Part print with two shaded views. Sizes in mm from the minimum x, y, z corner. Round coordinates to 2 decimals unless told otherwise and drop trailing zeros. Loops run counter-clockwise (first coordinate to the right, second up) from the corner with the lowest first, then second, coordinate; pieces in that order, holes last. Notation, with made-up numbers: (66, -0.5) -> (82, -0.5) arc R32 ccw to (82, 35.5) -> close; hole circle Ø1 at (88, 25). An arc over 180 degrees is marked (long way). Answer as a JSON object with one key per item and string values. Group by question number.
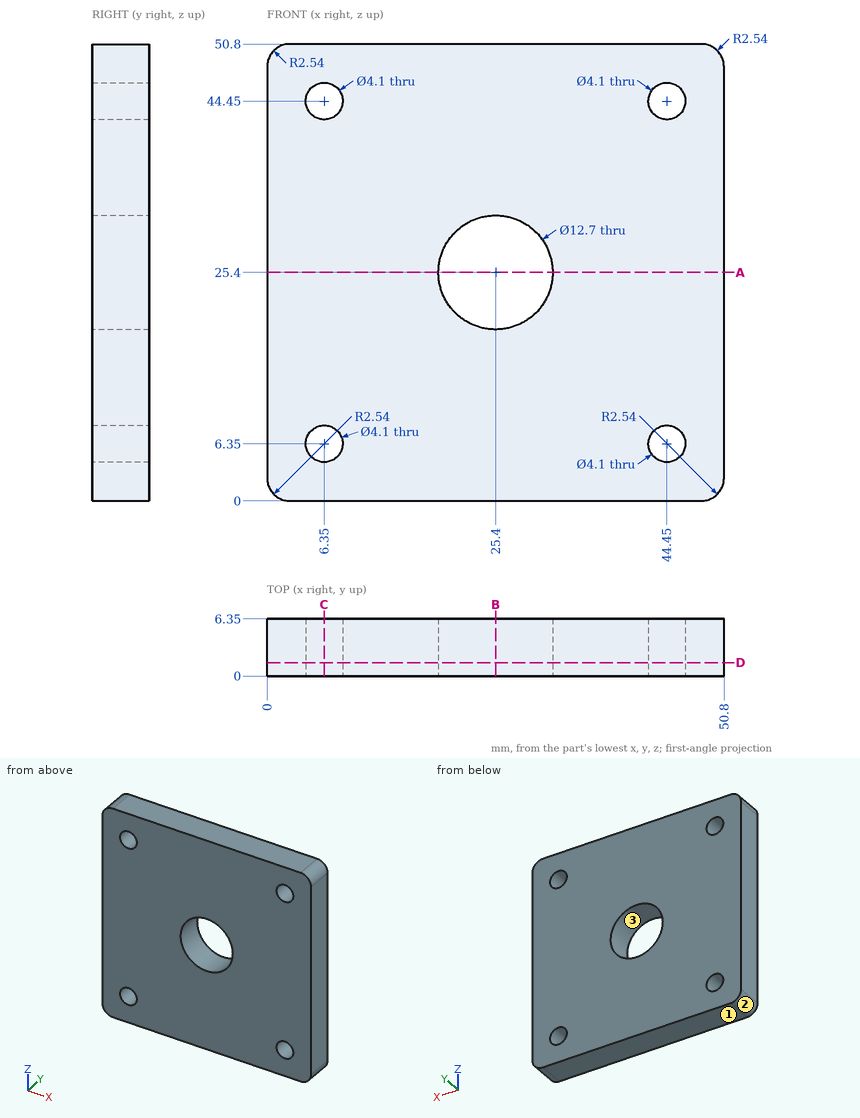
Item 1: Band-saw the part on A-A, the plane z = 25.4. List the corners of the cut face in (x, y).
Item 2: Drill centre lines: line 1 (X direction, y = 1.5, z = 6.35); line 2 (X direction, y = 3.75, z = 25.4); line 3 (Z direction, x = 43.5, y = 3). Where is each one in solid material? Low to high.
Item 3: Band-saw the part on D-D, the plane y = 1.5. List the corners of the cut face in (x, z), plus the area to 3 significant figures.
Item 4: Band-saw the part on B-B, the plane x = 25.4. List the corners of the cut face in (y, z), plus the area to 3 significant figures.
Item 5: Band-saw the part on C-C, the plane x = 6.35. List the corners of the cut face in (y, z), plus the area to 3 significant figures.
Item 6: Two-plate mould, pull along X, no slides. Class the marked faces 1, 2 and 3: pulls with the +X half, pulls with the -X half, needs draft (parallel to the pull), parting line crosses it, or undercut.
Entries:
{
 "1": {"outline": "(0, 0) -> (19.05, 0) -> (19.05, 6.35) -> (0, 6.35) -> close; (31.75, 0) -> (50.8, 0) -> (50.8, 6.35) -> (31.75, 6.35) -> close"},
 "2": {"line 1": "0 to 4.3, 8.4 to 42.4, 46.5 to 50.8", "line 2": "0 to 19.05, 31.75 to 50.8", "line 3": "0 to 4.53, 8.17 to 42.63, 46.27 to 50.8"},
 "3": {"outline": "(0, 2.54) arc R2.54 ccw to (2.54, 0) -> (48.26, 0) arc R2.54 ccw to (50.8, 2.54) -> (50.8, 48.26) arc R2.54 ccw to (48.26, 50.8) -> (2.54, 50.8) arc R2.54 ccw to (0, 48.26) -> close; hole circle Ø4.1 at (6.35, 6.35); hole circle Ø4.1 at (6.35, 44.45); hole circle Ø12.7 at (25.4, 25.4); hole circle Ø4.1 at (44.45, 6.35); hole circle Ø4.1 at (44.45, 44.45)", "area": "2,400 mm²"},
 "4": {"outline": "(0, 0) -> (6.35, 0) -> (6.35, 19.05) -> (0, 19.05) -> close; (0, 31.75) -> (6.35, 31.75) -> (6.35, 50.8) -> (0, 50.8) -> close", "area": "242 mm²"},
 "5": {"outline": "(0, 0) -> (6.35, 0) -> (6.35, 4.3) -> (0, 4.3) -> close; (0, 8.4) -> (6.35, 8.4) -> (6.35, 42.4) -> (0, 42.4) -> close; (0, 46.5) -> (6.35, 46.5) -> (6.35, 50.8) -> (0, 50.8) -> close", "area": "271 mm²"},
 "6": {"face 1": "needs draft", "face 2": "pulls with the -X half", "face 3": "undercut"}
}
